Job drawing, mm, ordinate dimensions from the low corner. One solid piece. A direction names the side the tool comes from. Give positions to 0.01 mm unless a question says otherwise; leave off trailing zeros. Write each loop counter-clockwise with the first axis right and the second up, starting at its lowest first coordinate (ties: lowest second). Pieces come first, ordered by that corner, then holes. Notation, with made-up numbers: (75, 82) - (88, 82) arc R14 ccw to (88, 99) - close; hole circle Ø2 at (-30.5, 54.25). An arc over 180 degrees is marked (long way). Answer as a JSON object with one key per item and string values.
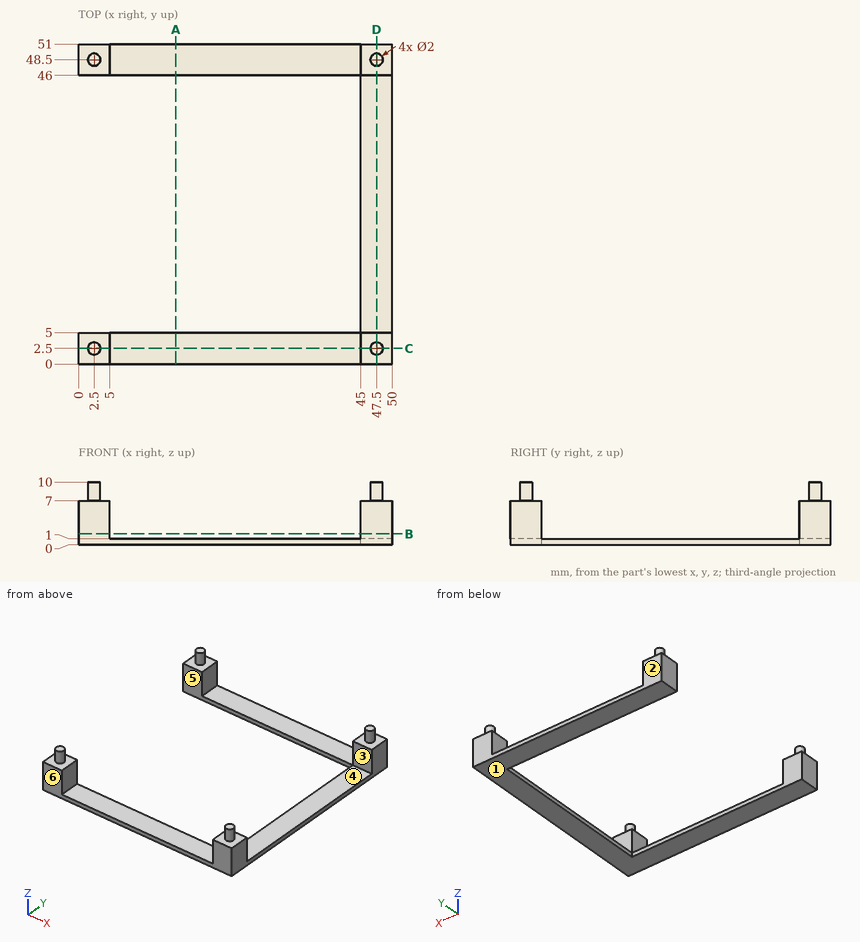
Item 1: Which spindle directions (+Z, -Z, +X, -X, +Y, -Y) get a long thin tool onto all of the face, cutting with end or side? Do the marked faces 4, 5 and 6. Say none if no direction does.
Entries:
{"face 4": "+Z, +X, -X", "face 5": "+Z, -Z, -X", "face 6": "+Z, -Z, +X, -X, -Y"}
Item 2: Flat gauge pins, fed straight in: P1, Ø4, axis at x = 22.5, y = 49, coming from the +Z side; P2, Ø0.8, axis at y = 18, z = 0.5, coming from the -X side. Where does each tip first touch, or does it go through?
Entries:
{"P1": "z = 1", "P2": "x = 45"}
Item 3: Cut at D-D (x = 47.5). Give the cut face in (y, z).
Entries:
{"outline": "(0, 0) - (51, 0) - (51, 7) - (49.5, 7) - (49.5, 10) - (47.5, 10) - (47.5, 7) - (46, 7) - (46, 1) - (5, 1) - (5, 7) - (3.5, 7) - (3.5, 10) - (1.5, 10) - (1.5, 7) - (0, 7) - close"}
Item 4: Mould opens along Y. For the marked faces 1, 2 and 3 say: +Y half, -Y half, draft (parallel to the pull), parting line (faces both ways), or undercut.
Entries:
{"face 1": "draft", "face 2": "+Y half", "face 3": "undercut"}
Item 5: Probe line 1 (Y direction, x = 10, z = 0.75); line 2 (Z direction, x = 18, y = 47). List the from-to ranges inside material, lowest first. Write a range as from..to.
Entries:
{"line 1": "0..5, 46..51", "line 2": "0..1"}
Item 6: Cut at B-B (z = 1.75). Give the cut face in (x, y), and give its area (3 significant figures).
Entries:
{"outline": "(0, 0) - (5, 0) - (5, 5) - (0, 5) - close; (0, 46) - (5, 46) - (5, 51) - (0, 51) - close; (45, 0) - (50, 0) - (50, 5) - (45, 5) - close; (45, 46) - (50, 46) - (50, 51) - (45, 51) - close", "area": "100 mm2"}
Item 7: Cut at A-A (x = 15.5). Give the cut face in (y, z).
Entries:
{"outline": "(0, 0) - (5, 0) - (5, 1) - (0, 1) - close; (46, 0) - (51, 0) - (51, 1) - (46, 1) - close"}
Item 8: Cut at C-C (y = 2.5). Give the cut face in (x, z), and give its area (3 significant figures).
Entries:
{"outline": "(0, 0) - (50, 0) - (50, 7) - (48.5, 7) - (48.5, 10) - (46.5, 10) - (46.5, 7) - (45, 7) - (45, 1) - (5, 1) - (5, 7) - (3.5, 7) - (3.5, 10) - (1.5, 10) - (1.5, 7) - (0, 7) - close", "area": "122 mm2"}
